Model file for the job. Use its own axes, mm. Round coordinates to 2 decimals unless told otherwise and drop trailing zeros. Loops run counter-clockwise (first coordinate to the right, second up) from the corner with the lowest first, then second, coordinate; pieces in that order, holes last. Notation, with made-up numbers: (-2.5, 49) - (2.5, 49) arc R10 ccw to (2.5, 65) - close; hole circle Ø10 at (77, -37.75). An arc over 180 degrees is marked (long way). Use one line per item in the form item = value.
from build123d import *

# Parameters (mm, degrees)
F0_W     = 100.5
F0_H     = 5
F0_R     = 1
F1_DEPTH = 1
F2_W     = 3.3293967307
F2_H     = 2
F3_DEPTH = 25
F4_R     = 0.99999


# Not quite as in the source:
# - a fillet or chamfer is up to 0.001 mm smaller than in the source, because OpenCascade refuses the exact size


with BuildPart() as f1:
    # F0 (on Front) → F1 (new body)
    with BuildSketch(Plane.XZ):
        Rectangle(F0_W, F0_H)
        with Locations((-47.75, 0)):
            Circle(F0_R, mode=Mode.SUBTRACT)
        with Locations((47.75, 0)):
            Circle(F0_R, mode=Mode.SUBTRACT)
    extrude(amount=F1_DEPTH)

    # F2 (on face) → F3 (cut)
    with BuildSketch(Plane.XZ.offset(1)):
        with Locations((-47.75, 0)):
            Rectangle(F2_W, F2_H)
    extrude(amount=-F3_DEPTH, mode=Mode.SUBTRACT)

    # F4 (radius 1 in the source; OpenCascade refuses exactly that, so slightly less here)
    f4_edges = [f1.edges().sort_by_distance(p)[0] for p in [
        (-46.085302, -0.5, 1),
        (-46.085302, -0.5, -1),
        (-49.414698, -0.5, 1),
        (-49.414698, -0.5, -1),
    ]]
    fillet(f4_edges, radius=F4_R)


solid = f1.part
1. Cut at A-A, the plane x = 47.75. Give the cut face in (y, z), plus the area to 3 significant figures.
Geometry check:
outline = (-1, -2.5) - (0, -2.5) - (0, -1) - (-1, -1) - close; (-1, 1) - (0, 1) - (0, 2.5) - (-1, 2.5) - close
area = 3.00 mm^2
2. Cut at B-B, the plane y = -0.15. Give the number of separate pieces and of enclosed holes in the cut face, plus the area to 3 significant figures.
Geometry check:
separate_pieces = 1
enclosed_holes = 2
area = 494 mm^2
3. Flat gauge pins, fed straight in: pin 1 (2 mm diameter, centred on x = -30, z = -1, fed in from +Y); pin 2 (1.8 mm diameter, centred on x = 47.75, z = 0, fed in from +Y). Where does each tip first touch, or does it go through?
Geometry check:
pin_1 = 0
pin_2 = through
4. Pull direction Z, two halves, no side cores. Call faces 1 (the flat face through (-1, 0, 0)), 2 (the cylindrical face through (48.704, -0.493, 0.3)): +Z half, -Z half, draft (parallel to the pull), parting line (faces both ways), or undercut.
Geometry check:
face_1 = draft
face_2 = undercut
5. Wall check: probe 1 along X at (y, z) = (-0.9, 0.15); probe 2 along Z at (x, y) = (47.75, -0.4); probe 3 along X at (y, z) = (-0.25, 0.7). Give the ranges that are in metal, low to high.
Geometry check:
probe_1 = -50.25 to -49.4, -46.1 to 46.76, 48.74 to 50.25
probe_2 = -2.5 to -1, 1 to 2.5
probe_3 = -50.25 to -49.13, -46.37 to 47.04, 48.46 to 50.25
